Print and shaded views of the part. All mm, measured from the part's lowest x, y and z. A direction names the side the tool comes from. Coordinates: 2 decimals unless noted, no trailing zeros. Order: outer loops, then holes, each group sorted by start corner. A loop starts at its lowest first (then second) coordinate and runs counter-clockwise, first axis right, second up. Notation, with made-up numbers: (51.5, 69.5) -> (88.5, 69.5) arc R19 cw to (88.5, 90.5) -> close; hole circle Ø11 at (4.5, 34). An arc over 180 degrees is marked (long way). Return JSON: item names as keys, results as strings. Group by question number.
1) Flat gauge pins, fed straight in: pin 1 (6 mm diameter, centred on x = 4, y = 10.75, fed in from -Z); pin 2 (6 mm diameter, centred on x = 10, z = 4, fed in from -Y); pin 3 (6.5 mm diameter, centred on x = 20.5, z = 2.5, fed in from +Y); pin 4 (1.5 mm diameter, centred on x = 29.5, y = 15.5, fed in from +Z). Where does each tip first touch, or does it go through?
2) Cut at C-C (x = 30). Write the cut outline in (y, z).
3) Which spindle directions (+Z, -Z, +X, -X, +Y, -Y) get a long thin tool onto all of the face, cutting with end or side? Do the marked faces 4, 5 and 6. Say none if no direction does.
4) Cut at A-A (y = 20.25). Write the cut outline in (x, z), and give its area (3 significant figures).
5) Pull direction Z, two halves, no side cores. Call the marked faces 1, 2 and 3: +Z half, -Z half, draft (parallel to the pull), parting line (faces both ways), or undercut.
6) Cut at D-D (y = 4.75). Write the cut outline in (x, z), and give its area (3 significant figures).
7) Probe line 1 (X direction, y = 2.65, z = 4); line 2 (Y direction, x = 4, z = 17.25); line 3 (X direction, y = 21.75, z = 16.5). List the from-to ranges inside material, lowest first.
8) Cut at B-B (z = 26). Write the cut outline in (x, y).
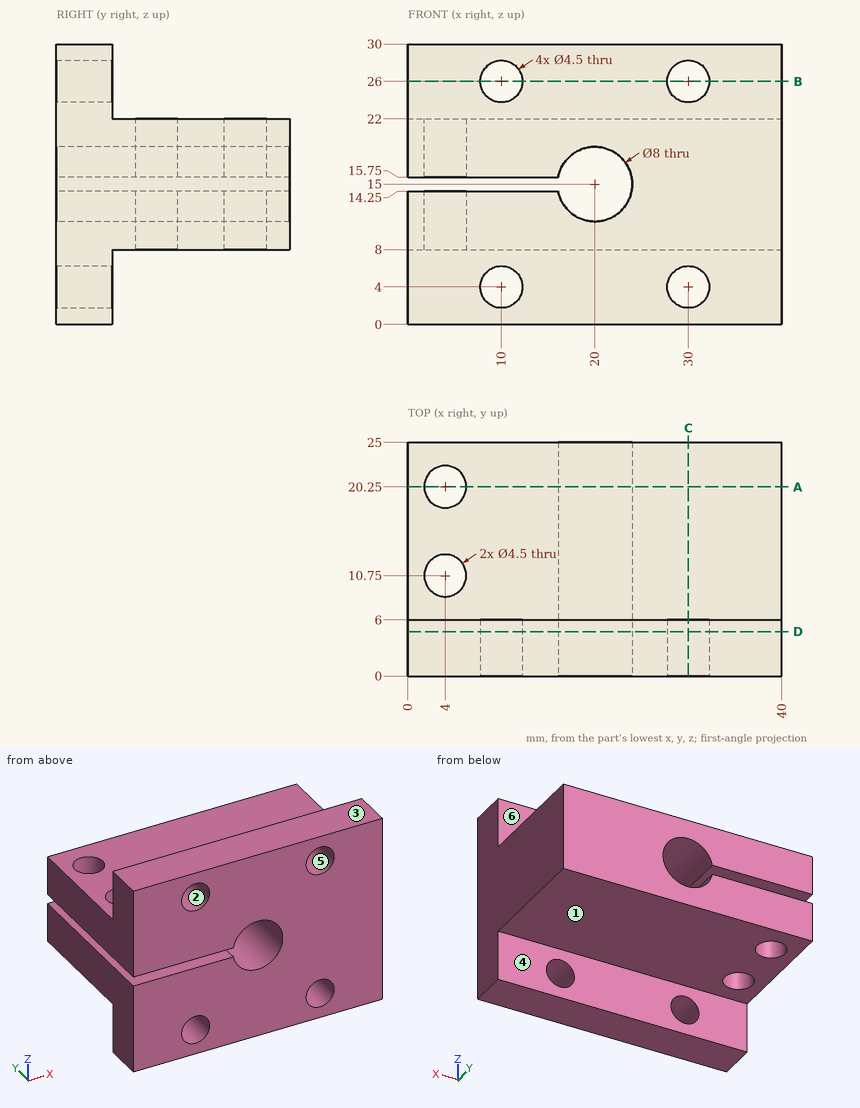
Answers below:
{
 "1": {"pin 1": "stops at z = 8", "pin 2": "stops at y = 0", "pin 3": "stops at y = 6", "pin 4": "stops at z = 22"},
 "2": {"outline": "(0, 0) -> (6, 0) -> (6, 1.75) -> (0, 1.75) -> close; (0, 6.25) -> (6, 6.25) -> (6, 8) -> (25, 8) -> (25, 22) -> (6, 22) -> (6, 23.75) -> (0, 23.75) -> close; (0, 28.25) -> (6, 28.25) -> (6, 30) -> (0, 30) -> close"},
 "3": {"face 4": "-Z, +X, -X, +Y", "face 5": "+Y, -Y", "face 6": "+Z, +X, -X, +Y"},
 "4": {"outline": "(0, 8) -> (1.75, 8) -> (1.75, 14.25) -> (0, 14.25) -> close; (0, 15.75) -> (1.75, 15.75) -> (1.75, 22) -> (0, 22) -> close; (6.25, 8) -> (40, 8) -> (40, 22) -> (6.25, 22) -> (6.25, 15.75) -> (16.07, 15.75) arc R4 cw (long way) to (16.07, 14.25) -> (6.25, 14.25) -> close", "area": "429 mm^2"},
 "5": {"face 1": "-Z half", "face 2": "undercut", "face 3": "+Z half"},
 "6": {"outline": "(0, 0) -> (40, 0) -> (40, 30) -> (0, 30) -> (0, 15.75) -> (16.07, 15.75) arc R4 cw (long way) to (16.07, 14.25) -> (0, 14.25) -> close; hole circle Ø4.5 at (10, 4); hole circle Ø4.5 at (10, 26); hole circle Ø4.5 at (30, 4); hole circle Ø4.5 at (30, 26)", "area": "1,060 mm^2"},
 "7": {"line 1": "x = 0 to 7.75, 12.25 to 27.75, 32.25 to 40", "line 2": "y = 0 to 8.5, 13 to 18, 22.5 to 25", "line 3": "x = 0 to 2.32, 5.68 to 16.29, 23.71 to 40"},
 "8": {"outline": "(0, 0) -> (7.75, 0) -> (7.75, 6) -> (0, 6) -> close; (12.25, 0) -> (27.75, 0) -> (27.75, 6) -> (12.25, 6) -> close; (32.25, 0) -> (40, 0) -> (40, 6) -> (32.25, 6) -> close"}
}
